Autodesk Inventor part; units mm, degrees
ref_plane "YZ Plane" through (0, 0, 0) normal (1, 0, 0) x (0, 1, 0)
ref_plane "XZ Plane" through (0, 0, 0) normal (0, 1, 0) x (-1, 0, 0)
ref_plane "XY Plane" through (0, 0, 0) normal (0, 0, 1) x (1, 0, 0)
sketch "Sketch1" plane through (0, 0, 0) normal (0, 0, 1) x (1, 0, 0)
  line L0 (0, 0) -> (99, 0)
  line L1 (99, 0) -> (99, 45.4)
  line L2 (99, 45.4) -> (0, 45.4)
  line L3 (0, 45.4) -> (0, 0)
  circle A0 centre (3, 42.4) radius 1.5
  circle A1 centre (3, 3) radius 1.5
  circle A2 centre (96, 3) radius 1.5
  circle A3 centre (96, 42.4) radius 1.5
  dimension "d0" = 45.4
  dimension "d1" = 99
  dimension "d2" = 3
  dimension "d3" = 3
  dimension "d4" = 3
  dimension "d5" = 3
  dimension "d6" = 3
  dimension "d7" = 3
  dimension "d8" = 3
  dimension "d9" = 3
  dimension "d10" = 3
  dimension "d11" = 3
  dimension "d12" = 3
  dimension "d13" = 3
extrude "Extrusion1" add sketch "Sketch1" along normal blind 1.6
fillet "Fillet1" radius 3 4 edges at (0, 0, 0.8) (99, 0, 0.8) (99, 45.4, 0.8) (0, 45.4, 0.8)
equation "\"d7\" = d6"
equation "\"d8\" = d9"
equation "\"d9\" = d7"
equation "\"d10\" = d11"
equation "\"d11\" = d8"
equation "\"d12\" = d10"
equation "\"d13\" = d12"
properties part number "Refplate"
Could you check a few things on this model? Use its own coordinates, in mm. Give positions to 0.01 mm unless a question says otherwise; leave off trailing zeros. Answer as CSV lines item,"result". Start each with the question number.
(1) I'm going to push flat-ended pins straight in: pin 1 Ø5 at (x, y) = (3, 42.4) entering from +Z; pin 2 Ø1.8 at (x, y) = (96, 42.4) entering from -Z. Where does each tip first touch, or does it pass through?
(2) We'd pull the mould along X, two halves only. Please class faces 1 (the cylindrical face through (3.806, 1.735, 0.789)), 2 (the flat face through (49, 23, 0)), 3 (the cylindrical face through (0.9, 44.54, 0.81)), 4 (the cylindrical face through (96.806, 1.735, 0.789)): released by +X, released by -X, zero draft, split by the parting line, or undercut.
(3) I need wall thicknesses on probe 1 along Y at (x, z) = (3, 1.1); probe 2 along X at (y, z) = (43, 1). Which ranges of each line are inside material? Lowest first, please.
Computed:
1,pin 1,"stops at z = 1.6"
1,pin 2,"passes through"
2,face 1,"undercut"
2,face 2,"zero draft"
2,face 3,"released by -X"
2,face 4,"undercut"
3,probe 1,"y = 0 to 1.5, 4.5 to 40.9, 43.9 to 45.4"
3,probe 2,"x = 0.06 to 1.63, 4.37 to 94.63, 97.37 to 98.94"
